CAD build for the part. Positions are in the model's coordinates, mm. A direction names the side the tool comes from. Round coordinates to 2 decimals unless told otherwise and drop trailing zeros. Write each loop counter-clockwise with the first axis right and the second up, starting at its lowest first coordinate (ties: lowest second). Pieces come first, ordered by that corner, then holes. Notation, with made-up numbers: (19.5, 40.25) - (75.5, 40.25) arc R36 cw to (75.5, 76.25) - close; hole circle Ø6 at (82.25, 17.25). An arc over 180 degrees is marked (long way). Answer in a Markdown table with one row per item.
```python
from build123d import *

# Parameters (mm, degrees)
SKETCH1_W           = 57
SKETCH1_H           = 57
BOSS_EXTRUDE1_DEPTH = 13
BOSS_EXTRUDE2_DEPTH = 30
SKETCH3_R           = 2.75
CUT_EXTRUDE1_DEPTH  = 57
SKETCH4_R           = 4.75
CUT_EXTRUDE6_DEPTH  = 54
SKETCH5_R           = 2.5
CUT_EXTRUDE7_DEPTH  = 5
SKETCH6_R           = 2.75
CUT_EXTRUDE8_DEPTH  = 14
SKETCH7_R           = 4.75
CUT_EXTRUDE9_DEPTH  = 5
FILLET1_R           = 3


with BuildPart() as part:
    # Sketch1 → Boss-Extrude1 (new body)
    with BuildSketch(Plane(origin=(0, 0, 0), x_dir=(1, 0, 0), z_dir=(0, 1, 0))):
        Rectangle(SKETCH1_W, SKETCH1_H)
    extrude(amount=BOSS_EXTRUDE1_DEPTH)

    # Sketch2 → Boss-Extrude2 (add)
    with BuildSketch(Plane(origin=(0, 13, 0), x_dir=(1, 0, 0), z_dir=(0, 1, 0))):
        with BuildLine():
            Line((0, 20), (-28.5, 20))
            Line((-28.5, 20), (-28.5, 28.5))
            Line((-28.5, 28.5), (28.5, 28.5))
            Line((28.5, 28.5), (28.5, -28.5))
            Line((28.5, -28.5), (-28.5, -28.5))
            Line((-28.5, -28.5), (-28.5, -20))
            Line((-28.5, -20), (0, -20))
            ThreePointArc((0, -20), (20, 0), (0, 20))
        make_face()
    extrude(amount=BOSS_EXTRUDE2_DEPTH)

    # Sketch3 → Cut-Extrude1 (cut)
    with BuildSketch(Plane.ZY.offset(28.5)):
        with Locations((0, 18)):
            Circle(SKETCH3_R)
        with Locations((0, 38)):
            Circle(SKETCH3_R)
    extrude(amount=-CUT_EXTRUDE1_DEPTH, mode=Mode.SUBTRACT)

    # Sketch4 → Cut-Extrude6 (cut)
    with BuildSketch(Plane.ZY.offset(28.5)):
        with Locations((0, 38)):
            Circle(SKETCH4_R)
        with Locations((0, 18)):
            Circle(SKETCH4_R)
    extrude(amount=-CUT_EXTRUDE6_DEPTH, mode=Mode.SUBTRACT)

    # Sketch5 → Cut-Extrude7 (cut)
    with BuildSketch(Plane(origin=(0, 43, 0), x_dir=(1, 0, 0), z_dir=(0, 1, 0))):
        with Locations((-23.57, 23.57)):
            Circle(SKETCH5_R)
        with Locations((23.57, 23.57)):
            Circle(SKETCH5_R)
        with Locations((23.57, -23.57)):
            Circle(SKETCH5_R)
        with Locations((-23.57, -23.57)):
            Circle(SKETCH5_R)
    extrude(amount=-CUT_EXTRUDE7_DEPTH, mode=Mode.SUBTRACT)

    # Sketch6 → Cut-Extrude8 (cut, through all)
    with BuildSketch(Plane(origin=(0, 13, 0), x_dir=(1, 0, 0), z_dir=(0, 1, 0))):
        with Locations((-18.5, 8.5)):
            Circle(SKETCH6_R)
        with Locations((8.5, 8.5)):
            Circle(SKETCH6_R)
    extrude(amount=-CUT_EXTRUDE8_DEPTH, mode=Mode.SUBTRACT)

    # Sketch7 → Cut-Extrude9 (cut)
    with BuildSketch(Plane(origin=(0, 13, 0), x_dir=(1, 0, 0), z_dir=(0, 1, 0))):
        with Locations((-18.5, 8.5)):
            Circle(SKETCH7_R)
        with Locations((8.5, 8.5)):
            Circle(SKETCH7_R)
    extrude(amount=-CUT_EXTRUDE9_DEPTH, mode=Mode.SUBTRACT)

    # Fillet1
    fillet1_edges = [part.edges().sort_by_distance(p)[0] for p in [
        (-28.5, 28, -20),
        (-28.5, 28, 20),
        (-28.5, 21.5, -28.5),
        (-28.5, 21.5, 28.5),
    ]]
    fillet(fillet1_edges, radius=FILLET1_R)


solid = part.part
```
Q1. Saw through at B-B on z = 0. List the corners of the cut face in (x, y).
Computed:
| item | result |
|---|---|
| outline | (-28.5, 0) - (28.5, 0) - (28.5, 15.25) - (25.5, 15.25) - (25.5, 13.25) - (20, 13.25) - (20, 13) - (-28.5, 13) - close; (20, 22.75) - (25.5, 22.75) - (25.5, 20.75) - (28.5, 20.75) - (28.5, 35.25) - (25.5, 35.25) - (25.5, 33.25) - (20, 33.25) - close; (20, 42.75) - (25.5, 42.75) - (25.5, 40.75) - (28.5, 40.75) - (28.5, 43) - (20, 43) - close |
Q2. 3-axis set-ups, long thin cutter, end or side, ignore diameter. For faces 1 (the flat face through (24, 38, -24)), 2 (the flat face through (-28.5, 12, 6)), 3 (the flat face through (-13, 28, 20)): which of +Z, -Z, +X, -X, +Y, -Y reach the whole face in a straight line?
Computed:
| item | result |
|---|---|
| face 1 | +Y |
| face 2 | +Z, -Z, -X, +Y, -Y |
| face 3 | -X, +Y |
Q3. Saw through at A-A on y = 18. List the corners of the cut face in (x, z), then the cut area to 3 significant figures.
Computed:
| item | result |
|---|---|
| outline | (-28.5, -25.5) arc R3 ccw to (-25.5, -28.5) - (28.5, -28.5) - (28.5, -2.75) - (25.5, -2.75) - (25.5, -4.75) - (19.43, -4.75) arc R20 cw to (0, -20) - (-25.5, -20) arc R3 ccw to (-28.5, -23) - close; (-28.5, 23) arc R3 ccw to (-25.5, 20) - (0, 20) arc R20 cw to (19.43, 4.75) - (25.5, 4.75) - (25.5, 2.75) - (28.5, 2.75) - (28.5, 28.5) - (-25.5, 28.5) arc R3 ccw to (-28.5, 25.5) - close |
| area | 1,400 mm2 |
Q4. Drill centre lines: line 1 (X direction, y = 2.5, z = -8.5); line 2 (X direction, y = 39.7, z = 23.57); line 3 (Z direction, x = 8.5, y = 5.25). Where is each one in solid material? Low to high.
Computed:
| item | result |
|---|---|
| line 1 | x = -28.5 to -21.25, -15.75 to 5.75, 11.25 to 28.5 |
| line 2 | x = -28.5 to -26.07, -21.07 to 21.07, 26.07 to 28.5 |
| line 3 | z = -28.5 to -11.25, -5.75 to 28.5 |
Q5. Saw through at C-C on y = 39. List the corners of the cut face in (x, z).
Computed:
| item | result |
|---|---|
| outline | (-28.5, -25.5) arc R3 ccw to (-25.5, -28.5) - (28.5, -28.5) - (28.5, -2.56) - (25.5, -2.56) - (25.5, -4.64) - (19.45, -4.64) arc R20 cw to (0, -20) - (-25.5, -20) arc R3 ccw to (-28.5, -23) - close; (-28.5, 23) arc R3 ccw to (-25.5, 20) - (0, 20) arc R20 cw to (19.45, 4.64) - (25.5, 4.64) - (25.5, 2.56) - (28.5, 2.56) - (28.5, 28.5) - (-25.5, 28.5) arc R3 ccw to (-28.5, 25.5) - close; hole circle Ø5 at (-23.57, -23.57); hole circle Ø5 at (-23.57, 23.57); hole circle Ø5 at (23.57, -23.57); hole circle Ø5 at (23.57, 23.57) |
Q6. Saw through at D-D on x = 23.57. List the corners of the cut face in (y, z).
Computed:
| item | result |
|---|---|
| outline | (0, -28.5) - (43, -28.5) - (43, -26.07) - (38, -26.07) - (38, -21.07) - (43, -21.07) - (43, 21.07) - (38, 21.07) - (38, 26.07) - (43, 26.07) - (43, 28.5) - (0, 28.5) - close; hole circle Ø9.5 at (18, 0); hole circle Ø9.5 at (38, 0) |
Q7. Flat gauge pins, fed straight in: pin 1 (8.5 mm diameter, centred on y = 18, z = 0, fed in from -X); pin 2 (5 mm diameter, centred on x = 7.5, z = -9, fed in from +Y); pin 3 (2.5 mm diameter, centred on x = 23.5, z = 23.5, fed in from +Y). Where does each tip first touch, or does it go through?
Computed:
| item | result |
|---|---|
| pin 1 | stops at x = 25.5 |
| pin 2 | stops at y = 8 |
| pin 3 | stops at y = 38 |
Q8. Pull direction Y, two halves, no side cores. Call faces 4 (the cylindrical face through (22.414, 38.209, -4.745)), 5 (the flat face through (25.5, 35, 0)), 6 (the cylindrical face through (-23.9, 40.53, -26.05)), 7 (the flat face through (-16, 8, -6)): released by +Y, released by -Y, zero draft, split by the parting line, or undercut.
Computed:
| item | result |
|---|---|
| face 4 | undercut |
| face 5 | undercut |
| face 6 | zero draft |
| face 7 | released by +Y |
